Geometry: final body of the model. Coordinates: model frame, mm. Round coordinates to 2 decimals unless told otherwise and drop trailing zeros. Order: outer loops, then holes, each group sorted by start corner. A loop starts at its lowest first (then second) coordinate and runs counter-clockwise, first axis right, second up. Notation, with made-up numbers: M 42,-29.5 L 99,-29.5 A26 ccw 99,-8.5 Z; hole C 82.25,64 d3. An arc over 180 degrees is marked long. Put each result on its own line as item: value. Start each with the question number.
1) Section A-A, the plane z = 1.55. Return loops of the section in (x, y), then the cut area to 3 significant figures.
2) Material intervals for probe 1 along Y at (x, z) = (0, 1); probe 2 along Y at (x, z) = (-12, 1.5); probe 3 along X at (y, z) = (-7, 2.15), sorted ascending. Write a range as [from, to].
3) First-contact query: P1, Ø1, axis at x = -4, z = 0, coming from the +Y side; P2, Ø1.5, axis at x = -2, z = 0, coming from the +Y side. Flat tips, straight axial feed; report the tip coordinate or a pass-through.
from build123d import *

# Parameters (mm, degrees)
F0_R     = 19.05
F1_DEPTH = 2.5
F2_R     = 6.375
F2_R_2   = 6.35
F3_DEPTH = 0.5


with BuildPart() as f1:
    # F0 (on Top) → F1 (new body)
    with BuildSketch(Plane.XY):
        Circle(F0_R)
    extrude(amount=F1_DEPTH)

    # F2 (on face) → F3 (cut)
    with BuildSketch(Plane.XY.offset(2.5)):
        Circle(F2_R)
        Circle(F2_R_2, mode=Mode.SUBTRACT)
    extrude(amount=-F3_DEPTH, mode=Mode.SUBTRACT)

    # F4 (on Front) → F5 (revolve)
    with BuildSketch(Plane.XZ):
        Polygon((0, -0.5), (0, 0), (-19.05, 0), (-17, -0.5), align=None)
    revolve(axis=Axis((0, 0, -0.25), (0, 0, -1)))


solid = f1.part
Result sheet:
1. outline: C 0,0 d38.1
1. area: 1,140 mm2
2. probe 1: y = [-19.05, 19.05]
2. probe 2: y = [-14.8, 14.8]
2. probe 3: x = [-17.72, 17.72]
3. P1: stops at y = 18.73
3. P2: stops at y = 19.01
